```python
from build123d import *

# Parameters (mm, degrees)
SKETCH_W    = 87.4
SKETCH_H    = 42.4
SKETCH_R    = 1.8
SKETCH_W_2  = 76.6
SKETCH_H_2  = 21.8
PAD_DEPTH   = 3
FILLET_R    = 4
FILLET001_R = 1


with BuildPart() as part:
    # Sketch → Pad (new body)
    with BuildSketch(Plane.XY):
        Rectangle(SKETCH_W, SKETCH_H)
        with Locations((-18.2, 17.2)):
            Circle(SKETCH_R, mode=Mode.SUBTRACT)
        with Locations((-18.2, -17.2)):
            Circle(SKETCH_R, mode=Mode.SUBTRACT)
        with Locations((26.8, -17.2)):
            Circle(SKETCH_R, mode=Mode.SUBTRACT)
        with Locations((26.8, 17.2)):
            Circle(SKETCH_R, mode=Mode.SUBTRACT)
        Rectangle(SKETCH_W_2, SKETCH_H_2, mode=Mode.SUBTRACT)
    extrude(amount=PAD_DEPTH)

    # Fillet
    fillet_edges = [part.edges().sort_by_distance(p)[0] for p in [
        (43.7, -21.2, 1.5),
        (-43.7, -21.2, 1.5),
        (43.7, 21.2, 1.5),
        (-43.7, 21.2, 1.5),
    ]]
    fillet(fillet_edges, radius=FILLET_R)

    # Fillet001
    fillet001_edges = [part.edges().sort_by_distance(p)[0] for p in [
        (38.3, 10.9, 1.5),
        (38.3, -10.9, 1.5),
        (-38.3, -10.9, 1.5),
        (-38.3, 10.9, 1.5),
    ]]
    fillet(fillet001_edges, radius=FILLET001_R)


solid = part.part
```
CAD build for the part. Positions are in the model's coordinates, mm. A direction names the side the tool comes from. Round coordinates to 2 decimals unless told otherwise and drop trailing zeros. Write each loop counter-clockwise with the first axis right and the second up, starting at its lowest first coordinate (ties: lowest second). Pieces come first, ordered by that corner, then holes. Notation, with made-up numbers: (21.25, 61.25) -> (63.25, 61.25) arc R11 cw to (63.25, 66.25) -> close; hole circle Ø10 at (7, 2). An arc over 180 degrees is marked (long way). Answer in a Markdown table with one row per item. Add a question column.
Item 1: Saw through at B-B, the plane z = 2.25. Write the cut outline in (x, y).
Item 2: Drill centre lines: line 1 (Y direction, x = -18.2, z = 1.2); line 2 (Y direction, x = -14, z = 1); line 3 (X direction, y = -3, z = 0.4). Where is each one in solid material? Low to high. Write a range as from..to.
Item 3: Which spindle directions (+Z, -Z, +X, -X, +Y, -Y) get a long thin tool onto all of the face, cutting with end or side? Do faces 1 (the face through (-42.559, 19.997, 1.521)), 2 (the face through (-1, -10.9, 1)). Say none if no direction does.
Item 4: Drop a flat-ended pin along its axis: pin 1 Ø8 at (x, y) = (-27, 3.5) entering from +Z (3 decimals). Give the stop position or say it passes through.
Item 5: Saw through at A-A, the plane x = -22.5. Write the cut outline in (y, z).
Item 6: Saw through at C-C, the plane x = 26.8. Write the cut outline in (y, z), then the cut area to 3 significant figures.
Item 7: Mould opens along X. For faces 3 (the face through (43.7, 0, 1)), 4 (the face through (-18.434, 18.985, 1.479)), 5 (the face through (-42.559, -19.997, 1.521)) say: pulls with the +X half, pulls with the -X half, needs draft (parallel to the pull), parting line crosses it, or undercut.
Findings below:
| question | item | result |
|---|---|---|
| 1 | outline | (-43.7, -17.2) arc R4 ccw to (-39.7, -21.2) -> (39.7, -21.2) arc R4 ccw to (43.7, -17.2) -> (43.7, 17.2) arc R4 ccw to (39.7, 21.2) -> (-39.7, 21.2) arc R4 ccw to (-43.7, 17.2) -> close; hole (-38.3, -9.9) arc R1 ccw to (-37.3, -10.9) -> (37.3, -10.9) arc R1 ccw to (38.3, -9.9) -> (38.3, 9.9) arc R1 ccw to (37.3, 10.9) -> (-37.3, 10.9) arc R1 ccw to (-38.3, 9.9) -> close; hole circle Ø3.6 at (-18.2, -17.2); hole circle Ø3.6 at (-18.2, 17.2); hole circle Ø3.6 at (26.8, -17.2); hole circle Ø3.6 at (26.8, 17.2) |
| 2 | line 1 | y = -21.2..-19, -15.4..-10.9, 10.9..15.4, 19..21.2 |
| 2 | line 2 | y = -21.2..-10.9, 10.9..21.2 |
| 2 | line 3 | x = -43.7..-38.3, 38.3..43.7 |
| 3 | face 1 | +Z, -Z, -X, +Y |
| 3 | face 2 | +Z, -Z |
| 4 | pin 1 | passes through |
| 5 | outline | (-21.2, 0) -> (-10.9, 0) -> (-10.9, 3) -> (-21.2, 3) -> close; (10.9, 0) -> (21.2, 0) -> (21.2, 3) -> (10.9, 3) -> close |
| 6 | outline | (-21.2, 0) -> (-19, 0) -> (-19, 3) -> (-21.2, 3) -> close; (-15.4, 0) -> (-10.9, 0) -> (-10.9, 3) -> (-15.4, 3) -> close; (10.9, 0) -> (15.4, 0) -> (15.4, 3) -> (10.9, 3) -> close; (19, 0) -> (21.2, 0) -> (21.2, 3) -> (19, 3) -> close |
| 6 | area | 40.2 mm^2 |
| 7 | face 3 | pulls with the +X half |
| 7 | face 4 | undercut |
| 7 | face 5 | pulls with the -X half |
